from build123d import *

# Parameters (mm, degrees)
SKETCH1_W                     = 76
SKETCH1_H                     = 50
UAV_INTERFACE_TOP_DEPTH       = 6
SKETCH2_W                     = 10
SKETCH2_H                     = 50
SPOOL_AND_MOTOR_INSERTS_DEPTH = 80
SKETCH3_R                     = 17.3
MOTOR_CUTOUT_DEPTH            = 30


with BuildPart() as part:
    # Sketch1 → UAV Interface Top (new body)
    with BuildSketch(Plane(origin=(0, 0, 0), x_dir=(1, 0, 0), z_dir=(0, 1, 0))):
        with Locations((38, 25)):
            Rectangle(SKETCH1_W, SKETCH1_H)
    extrude(amount=-UAV_INTERFACE_TOP_DEPTH)

    # Sketch2 → Spool and Motor Inserts (add)
    with BuildSketch(Plane.XZ.offset(6)):
        with Locations((71, -25)):
            Rectangle(SKETCH2_W, SKETCH2_H)
    extrude(amount=SPOOL_AND_MOTOR_INSERTS_DEPTH)

    # Mirror1: part across plane


with BuildPart() as part_1:
    add(part.part)
    add(part.part.mirror(Plane(origin=(38, 0, 0), x_dir=(0, 0, 1), z_dir=(1, 0, 0))))

    # Sketch3 → Motor Cutout (cut)
    with BuildSketch(Plane(origin=(76, 0, 0), x_dir=(0, 0, -1), z_dir=(1, 0, 0))):
        with Locations((25, -56)):
            Circle(SKETCH3_R)
    extrude(amount=-MOTOR_CUTOUT_DEPTH, mode=Mode.SUBTRACT)


solid = part_1.part
Read the model definition and answer for the solid it produces. Units are mm, in the model's axes. A direction names the side the tool comes from. Coordinates: 2 decimals unless noted, no trailing zeros. Loops run counter-clockwise (first coordinate to the right, second up) from the corner with the lowest first, then second, coordinate; pieces in that order, holes last. Notation, with made-up numbers: (81.25, 75.25) -> (111.25, 75.25) arc R22 cw to (111.25, 82.25) -> close; hole circle Ø4 at (13, -7.75). An arc over 180 degrees is marked (long way). Answer in a Markdown table with one row per item.
Item 1: A cutting plane is placed at B-B on z = -25. Determine the outline of the cut face in (x, y), plus the area to 3 significant figures.
Returned:
| item | result |
|---|---|
| outline | (0, -86) -> (10, -86) -> (10, -6) -> (66, -6) -> (66, -38.7) -> (76, -38.7) -> (76, 0) -> (0, 0) -> close; (66, -86) -> (76, -86) -> (76, -73.3) -> (66, -73.3) -> close |
| area | 1,710 mm^2 |
Item 2: A cutting plane is placed at C-C on y = -56. Determine the outline of the cut face in (x, z), plus the area to 3 significant figures.
Returned:
| item | result |
|---|---|
| outline | (0, -50) -> (10, -50) -> (10, 0) -> (0, 0) -> close; (66, -50) -> (76, -50) -> (76, -42.3) -> (66, -42.3) -> close; (66, -7.7) -> (76, -7.7) -> (76, 0) -> (66, 0) -> close |
| area | 654 mm^2 |
Item 3: A cutting plane is placed at A-A on y = -13.5. Determine the outline of the cut face in (x, z), plus the area to 3 significant figures.
Returned:
| item | result |
|---|---|
| outline | (0, -50) -> (10, -50) -> (10, 0) -> (0, 0) -> close; (66, -50) -> (76, -50) -> (76, 0) -> (66, 0) -> close |
| area | 1,000 mm^2 |
Item 4: This flat-tipped pin is pushed along its axis until it touches: P1, Ø2, axis at x = 58.5, z = -42.5, coming from the -Y side. Where does it stop, or does it pass through?
Returned:
| item | result |
|---|---|
| P1 | stops at y = -6 |
Item 5: Straight lines are drawn through the part: line 1 along X through (y, z) = (-44.5, -12); line 2 along Y through (x, z) = (72.25, -25); line 3 along Y through (x, z) = (26.5, -43). For each, find the intervals that lie inside material, in ascending order. Write a range as [from, to].
Returned:
| item | result |
|---|---|
| line 1 | x = [0, 10], [66, 76] |
| line 2 | y = [-86, -73.3], [-38.7, 0] |
| line 3 | y = [-6, 0] |
Item 6: A cutting plane is placed at D-D on z = -5.5. Determine the outline of the cut face in (x, y), plus the area to 3 significant figures.
Returned:
| item | result |
|---|---|
| outline | (0, -86) -> (10, -86) -> (10, -6) -> (66, -6) -> (66, -86) -> (76, -86) -> (76, 0) -> (0, 0) -> close |
| area | 2,060 mm^2 |
Item 7: For faces 1 (the flat face through (37, 0, -25)), 2 (the flat face through (66, -37, -25)), determine the directions among +Z, -Z, +X, -X, +Y, -Y from which every point of the face is accessible in a straight line to the end or side of a thin tool.
Returned:
| item | result |
|---|---|
| face 1 | +Z, -Z, +X, -X, +Y |
| face 2 | +Z, -Z, -Y |
Item 8: For a pull along Z with two mould halves and no side action, classify faces 3 (the flat face through (5, -86, -25)), 4 (the cylindrical face through (71.07, -38.847, -22.748)), 5 (the flat face through (66.3, -33.2, -50)) as released by +Z, released by -Z, zero draft, split by the parting line, or undercut.
Returned:
| item | result |
|---|---|
| face 3 | zero draft |
| face 4 | undercut |
| face 5 | released by -Z |
